Part model, mm, in its own coordinate system. Round coordinates to 2 decimals unless told otherwise and drop trailing zeros. Write each loop counter-clockwise with the first axis right and the second up, starting at its lowest first coordinate (ties: lowest second). Pieces come first, ordered by that corner, then holes. Notation, with made-up numbers: (13.25, -17.75) -> (24.25, -17.75) arc R21 cw to (24.25, -3.75) -> close; hole circle Ø11 at (74, 9). An arc over 180 degrees is marked (long way). Return JSON: item names as keys, results as strings. Group by question number.
(1) Drill centre lines: L1, parallel to X at y = -9.5, z = 3.2; L2, parallel to X at y = 15, z = 1.9; L3, parallel to X at y = 9, z = 1.8. Where is each one in solid material? Low to high. Write a range as from..to.
(2) Saw through at A-A (x = -27.5). List the corners of the cut face in (y, z), plus the area to 3 significant figures.
(3) Saw through at B-B (z = 1.55). State how many separate pieces and enclosed holes the cut face has, plus the area to 3 significant figures.
(4) Drop flat-ended pins along their axis: pin 1 Ø1.2 at (x, z) = (54, 1) entering from +Y; pin 2 Ø2 at (x, z) = (50.5, 1) entering from -Y; pin 3 Ø2 at (x, z) = (50, 3) entering from -Y. Give the stop position or say it passes through.
from build123d import *

# Parameters (mm, degrees)
SKIZZE2_R                       = 12.5
AUFSATZ_LINEAR_AUSTRAGEN2_DEPTH = 4


with BuildPart() as part:
    # Skizze2 → Aufsatz-Linear austragen2 (new body)
    with BuildSketch(Plane.XY):
        with BuildLine():
            Line((-36.002800277, 29.622112019), (23.801047301, 29.622112019))
            add(Edge.make_bspline(
                [(23.801047301, 29.622112019), (39.324007896, 29.622112019), (44.325198534, 27.788269736)],
                knots=[0, 0, 0, 1, 1, 1], degree=2))
            ThreePointArc((44.325198534, 27.788269736), (47.84965812, 26.232437014), (51.145668645, 24.237757727))
            add(Edge.make_bspline(
                [(51.145668645, 24.237757727), (55.926029521, 20.907523335), (61.370340825, 13.799078949), (62.982460357, 7.357685339)],
                knots=[0, 0, 0, 0, 1, 1, 1, 1], degree=3))
            ThreePointArc((62.982460357, 7.357685339), (62.618871056, 5.641491574), (61.042300943, 4.872112019))
            Line((61.042300943, 4.872112019), (47.785287356, 4.872112019))
            Line((47.785287356, 4.872112019), (39.265024534, 7.815111963))
            ThreePointArc((39.265024534, 7.815111963), (18.497199723, -0.377887981), (39.265024534, -8.570887926))
            Line((39.265024534, -8.570887926), (47.785287356, -5.627887981))
            Line((47.785287356, -5.627887981), (61.042300943, -5.627887981))
            ThreePointArc((61.042300943, -5.627887981), (62.618871056, -6.397267536), (62.982460357, -8.113461302))
            add(Edge.make_bspline(
                [(51.145668645, -24.99353369), (55.926029521, -21.663299298), (61.370340825, -14.554854912), (62.982460357, -8.113461302)],
                knots=[0, 0, 0, 0, 1, 1, 1, 1], degree=3))
            ThreePointArc((51.145668645, -24.99353369), (47.84965812, -26.988212977), (44.325198534, -28.544045699))
            add(Edge.make_bspline(
                [(23.801047301, -30.377887981), (39.324007896, -30.377887981), (44.325198534, -28.544045699)],
                knots=[0, 0, 0, 1, 1, 1], degree=2))
            Line((23.801047301, -30.377887981), (-36.002800277, -30.377887981))
            ThreePointArc((-36.002800277, -30.377887981), (-66.002800277, -0.377887981), (-36.002800277, 29.622112019))
        make_face()
        with Locations((-36.002800277, -0.377887981)):
            Circle(SKIZZE2_R, mode=Mode.SUBTRACT)
        with BuildLine():
            Line((22.940850537, 17.278461205), (16.940850537, 17.278461205))
            ThreePointArc((16.940850537, 17.278461205), (14.840850537, 15.178461205), (16.940850537, 13.078461205))
            Line((16.940850537, 13.078461205), (22.940850537, 13.078461205))
            ThreePointArc((22.940850537, 13.078461205), (25.040850537, 15.178461205), (22.940850537, 17.278461205))
        make_face(mode=Mode.SUBTRACT)
        with BuildLine():
            Line((48.05354891, 13.078461205), (54.05354891, 13.078461205))
            ThreePointArc((54.05354891, 13.078461205), (56.15354891, 15.178461205), (54.05354891, 17.278461205))
            Line((54.05354891, 17.278461205), (48.05354891, 17.278461205))
            ThreePointArc((48.05354891, 17.278461205), (45.95354891, 15.178461205), (48.05354891, 13.078461205))
        make_face(mode=Mode.SUBTRACT)
        with BuildLine():
            Line((48.05354891, -17.984237167), (54.05354891, -17.984237167))
            ThreePointArc((54.05354891, -17.984237167), (56.10354891, -15.934237167), (54.05354891, -13.884237167))
            Line((54.05354891, -13.884237167), (48.05354891, -13.884237167))
            ThreePointArc((48.05354891, -13.884237167), (46.00354891, -15.934237167), (48.05354891, -17.984237167))
        make_face(mode=Mode.SUBTRACT)
        with BuildLine():
            Line((22.940850537, -13.834237167), (16.940850537, -13.834237167))
            ThreePointArc((16.940850537, -13.834237167), (14.840850537, -15.934237167), (16.940850537, -18.034237167))
            Line((16.940850537, -18.034237167), (22.940850537, -18.034237167))
            ThreePointArc((22.940850537, -18.034237167), (25.040850537, -15.934237167), (22.940850537, -13.834237167))
        make_face(mode=Mode.SUBTRACT)
        with BuildLine():
            ThreePointArc((-23.345588893, -13.035099365), (-21.119494216, -10.322595152), (-19.465356645, -7.227921421))
            ThreePointArc((-19.465356645, -7.227921421), (-16.721574418, -6.09140961), (-15.585062608, -8.835191837))
            ThreePointArc((-15.585062608, -8.835191837), (-17.627321845, -12.655990131), (-20.375740412, -16.004947846))
            ThreePointArc((-20.375740412, -16.004947846), (-23.345588893, -16.004947846), (-23.345588893, -13.035099365))
        make_face(mode=Mode.SUBTRACT)
        with BuildLine():
            ThreePointArc((-40.635661184, -17.667960272), (-37.17351629, -18.239562707), (-33.666381436, -18.124751))
            ThreePointArc((-33.666381436, -18.124751), (-31.310242223, -19.932680205), (-33.118171429, -22.288819418))
            ThreePointArc((-33.118171429, -22.288819418), (-37.448209433, -22.430570185), (-41.722701173, -21.724848742))
            ThreePointArc((-41.722701173, -21.724848742), (-43.207625414, -19.152884512), (-40.635661184, -17.667960272))
        make_face(mode=Mode.SUBTRACT)
        with BuildLine():
            ThreePointArc((-53.292872567, -5.010748889), (-52.05682235, -8.294855536), (-50.203825068, -11.274717561))
            ThreePointArc((-50.203825068, -11.274717561), (-50.591468081, -14.219158576), (-53.535909097, -13.831515562))
            ThreePointArc((-53.535909097, -13.831515562), (-55.823687864, -10.152468035), (-57.349761038, -6.097788878))
            ThreePointArc((-57.349761038, -6.097788878), (-55.864836797, -3.525824648), (-53.292872567, -5.010748889))
        make_face(mode=Mode.SUBTRACT)
        with BuildLine():
            ThreePointArc((-48.66001166, 12.279323402), (-50.886106337, 9.56681919), (-52.540243909, 6.472145458))
            ThreePointArc((-52.540243909, 6.472145458), (-55.284026135, 5.335633648), (-56.420537945, 8.079415874))
            ThreePointArc((-56.420537945, 8.079415874), (-54.378278708, 11.900214168), (-51.629860141, 15.249171883))
            ThreePointArc((-51.629860141, 15.249171883), (-48.66001166, 15.249171883), (-48.66001166, 12.279323402))
        make_face(mode=Mode.SUBTRACT)
        with BuildLine():
            ThreePointArc((-31.369939369, 16.912184309), (-34.832084263, 17.483786745), (-38.339219117, 17.368975037))
            ThreePointArc((-38.339219117, 17.368975037), (-40.69535833, 19.176904242), (-38.887429125, 21.533043455))
            ThreePointArc((-38.887429125, 21.533043455), (-34.557391121, 21.674794222), (-30.28289938, 20.96907278))
            ThreePointArc((-30.28289938, 20.96907278), (-28.797975139, 18.39710855), (-31.369939369, 16.912184309))
        make_face(mode=Mode.SUBTRACT)
        with BuildLine():
            ThreePointArc((-18.712727986, 4.254972926), (-16.140763756, 2.770048686), (-14.655839516, 5.342012915))
            ThreePointArc((-14.655839516, 5.342012915), (-16.181912689, 9.396692073), (-18.469691456, 13.0757396))
            ThreePointArc((-18.469691456, 13.0757396), (-21.414132472, 13.463382613), (-21.801775485, 10.518941598))
            ThreePointArc((-21.801775485, 10.518941598), (-19.948778203, 7.539079574), (-18.712727986, 4.254972926))
        make_face(mode=Mode.SUBTRACT)
    extrude(amount=AUFSATZ_LINEAR_AUSTRAGEN2_DEPTH)


solid = part.part
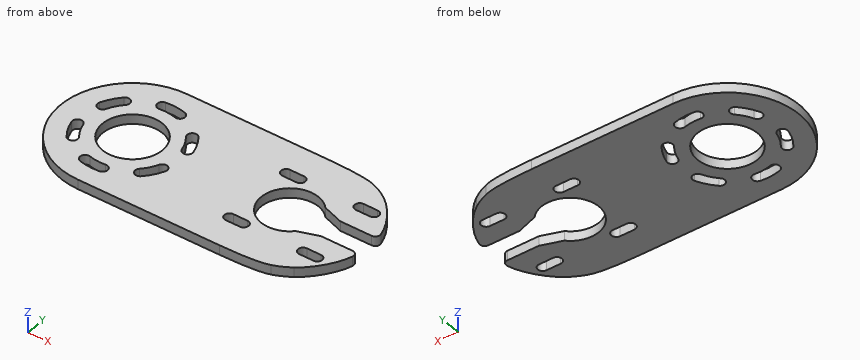
Computed values:
{
 "1": {"L1": "-64.58..-56.13, -51.4..-44.55, -27.46..-20.6, -15.87..22.7, 38.29..62.58", "L2": "-61.76..-51.88, -48.45..14.85, 25.03..45.96, 56.15..59.57", "L3": "-64.5..-56.01, -51.25..-44.27, -27.74..-20.76, -15.99..23.01, 37.98..62.5"},
 "2": {"outline": "(-30.38, 0) -> (-9.54, 0) -> (-9.54, 4) -> (-30.38, 4) -> close; (8.78, 0) -> (29.62, 0) -> (29.62, 4) -> (8.78, 4) -> close", "area": "167 mm2"},
 "3": {"separate pieces": "1", "enclosed holes": "11", "area": "5,390 mm2"},
 "4": {"pin 1": "y = 22.43", "pin 2": "y = -26.06", "pin 3": "y = -26.36"}
}
